from build123d import *

# Parameters (mm, degrees)
BOSS_EXTRUDE1_DEPTH      = 15
H_0_266_DIAMETER_HOLE1_D = 6.7564
SKETCH5_W                = 40
SKETCH5_H                = 16
SKETCH5_H_2              = 20.916111238
CUT_EXTRUDE1_DEPTH       = 243.332416321


with BuildPart() as part:
    # Sketch1 → Boss-Extrude1 (new, symmetric)
    with BuildSketch(Plane.XY):
        with BuildLine():
            Line((-225, 15), (225, 15))
            ThreePointArc((225, 15), (240, 0), (225, -15))
            Line((225, -15), (-225, -15))
            ThreePointArc((-225, -15), (-240, 0), (-225, 15))
        make_face()
    extrude(amount=BOSS_EXTRUDE1_DEPTH, both=True)

    # H (0.266) Diameter Hole1 (through all)
    with Locations(Plane.XY.offset(15)):
        with Locations((-225, 0), (225, 0)):
            Hole(H_0_266_DIAMETER_HOLE1_D / 2)

    # Sketch5 → Cut-Extrude1 (cut, through all)
    with BuildSketch(Plane(origin=(0, 15, 0), x_dir=(1, 0, 0), z_dir=(0, 1, 0))):
        with Locations((-237, 0)):
            Rectangle(SKETCH5_W, SKETCH5_H)
        with Locations((227, 18.458055619)):
            Rectangle(SKETCH5_W, SKETCH5_H_2)
        with Locations((227, -18.458055619)):
            Rectangle(SKETCH5_W, SKETCH5_H_2)
    extrude(amount=-CUT_EXTRUDE1_DEPTH, mode=Mode.SUBTRACT)


solid = part.part
Check sheet for the modelled part. Datum: model origin and axes. Units: mm. A direction names the side the tool comes from. Round coordinates to 2 decimals unless told otherwise and drop trailing zeros. Order: outer loops, then holes, each group sorted by start corner. A loop starts at its lowest first (then second) coordinate and runs counter-clockwise, first axis right, second up. Notation, with made-up numbers: M 52,-35 L 65,-35 A15 cw 65,-30 Z; hole C -13,37 d11. An arc over 180 degrees is marked long. One line per item, written item: value. Start each with the question number.
1. Access from +Z, -Z, +X, -X, +Y, -Y to the whole of each face (thin tool, end or side, straight path). Record for faces 1 (the cylindrical face through (-240, 0, -11)), 2 (the flat face through (-229, 0, -8)), 3 (the flat face through (220, 0, -8)).
2. Section check A-A on z = -0.25. Enter the section's corners in (x, y).
3. Release check for a two-part mould opening along Z. For faces 4 (the flat face through (-217, 0, 0)), 5 (the flat face through (220, 0, 8)), 6 (the cylindrical face through (240, 0, 0)) record: released by +Z, released by -Z, zero draft, split by the parting line, or undercut.
4. Scan lines: line 1 along Y through (x, z) = (225, -2.25); line 2 along X through (y, z) = (1.5, 12.5); line 3 along X through (y, z) = (10.5, -9.5). Record each from-to range of solid material in increasing order.
5. Gauge pin test, flat ends, axial feed: P1, Ø2, axis at y = -0.5, z = -12.5, coming from the +X side; P2, Ø3, axis at y = 11.5, z = 2.5, coming from the +X side; P3, Ø2, axis at y = 7.5, z = 3.5, coming from the +X side. Record the tip position at first contact, or that the pin passes through.
Results found:
1. face 1: +Z, -Z, -X
1. face 2: -X, +Y, -Y
1. face 3: -Z, +X, +Y, -Y
2. outline: M -217,-15 L 225,-15 A15 ccw 225,15 L -217,15 Z; hole C 225,0 d6.76
3. face 4: undercut
3. face 5: released by +Z
3. face 6: zero draft
4. line 1: -15 to -3.38, 3.38 to 15
4. line 2: -239.92 to -228.03, -221.97 to 207
4. line 3: -235.71 to 207
5. P1: x = 207
5. P2: x = 236.18
5. P3: x = 238.52
